Can you work these out from the model? Positions are in its coordinate system, mm. A direction names the side the tool comes from. Give positions to 0.01 mm unless a question says otherwise; leave off trailing zeros. Loops run counter-clockwise (first coordinate to the right, second up) from the corner with the lowest first, then second, coordinate; pieces in that order, holes last. Notation, with made-up numbers: M 79.25,18.25 L 109.25,18.25 A14 cw 109.25,29.25 Z; hole C 41.5,-12 d6. An arc over 180 degrees is marked long. Put each result on its own line as item: value. Start each with the question number.
1) For P1, Ø5, axis at y = 159.5, z = 3.5, coming from the -X side; P2, Ø2, axis at x = -6, z = -2.5, coming from the +Y side; P3, Ø1.5, axis at x = -5.5, y = 27.5, coming from the +Z side, each with a flat end and sliding along its axis, tell me the tip position at first contact or that it passes through.
2) Imagine slicing it at A-A (x = 0). Write out the boundary of the cut face in (y, z).
3) For faces 1 (the cylindrical face through (-2, 182, 0)), 2 (the flat face through (0, 0, 0)), 3 (the cylindrical face through (1.802, 73.95, 5.723)), which set-ups out of +Z, -Z, +X, -X, +Y, -Y let a thin tool reach every point of the face, with its end or its side?
4) Imagine slicing it at B-B (z = 0). Write out the boundary of the cut face in (x, y), then the cut area to 3 significant figures.
5) Imagine slicing it at C-C (y = 59). Write out the boundary of the cut face in (x, z), then the cut area to 3 significant figures.
6) Please list where these lines run through material, in increasing order: line 1 along Y through (x, z) = (3, 3.75); line 2 along Y through (x, z) = (0, 6.5); line 3 along X through (y, z) = (123, 0.5). Write a range as from..to.
from build123d import *

# Parameters (mm, degrees)
SKETCH1_R            = 6
ELECTRODE_BODY_DEPTH = 150
CAP_START            = 150
SKETCH2_R            = 8
CAP_DEPTH            = 25
CABLE_STUB_START     = 175
SKETCH3_R            = 2
CABLE_STUB_DEPTH     = 15
SKETCH4_R            = 2
PLATINUM_TIP_DEPTH   = 1.5


with BuildPart() as part:
    # Sketch1 → Electrode_Body (new body)
    with BuildSketch(Plane(origin=(0, 0, 0), x_dir=(1, 0, 0), z_dir=(0, 1, 0))):
        with Locations(Location((0, 0, 0), (0, 0, 270))):
            Circle(SKETCH1_R)
    extrude(amount=ELECTRODE_BODY_DEPTH)

    # Sketch2 → Cap (add)
    with BuildSketch(Plane(origin=(0, 0, 0), x_dir=(1, 0, 0), z_dir=(0, 1, 0)).offset(CAP_START)):
        with Locations(Location((0, 0, 0), (0, 0, 270))):
            Circle(SKETCH2_R)
    extrude(amount=CAP_DEPTH)

    # Sketch3 → Cable_Stub (add)
    with BuildSketch(Plane(origin=(0, 0, 0), x_dir=(1, 0, 0), z_dir=(0, 1, 0)).offset(CABLE_STUB_START)):
        with Locations(Location((0, 0, 0), (0, 0, 270))):
            Circle(SKETCH3_R)
    extrude(amount=CABLE_STUB_DEPTH)

    # Sketch4 → Platinum_Tip (add)
    with BuildSketch(Plane(origin=(0, 0, 0), x_dir=(1, 0, 0), z_dir=(0, 1, 0))):
        with Locations(Location((0, 0, 0), (0, 0, 270))):
            Circle(SKETCH4_R)
    extrude(amount=PLATINUM_TIP_DEPTH)


solid = part.part
Recorded:
1. P1: x = -7.94
1. P2: y = 175
1. P3: z = 3.67
2. outline: M 0,-6 L 150,-6 L 150,-8 L 175,-8 L 175,-2 L 190,-2 L 190,2 L 175,2 L 175,8 L 150,8 L 150,6 L 0,6 Z
3. face 1: +Y
3. face 2: +Z, -Z, +X, -X, -Y
3. face 3: -Y
4. outline: M -8,150 L -6,150 L -6,0 L 6,0 L 6,150 L 8,150 L 8,175 L 2,175 L 2,190 L -2,190 L -2,175 L -8,175 Z
4. area: 2,260 mm²
5. outline: C 0,0 d12
5. area: 113 mm²
6. line 1: 0..175
6. line 2: 150..175
6. line 3: -5.98..5.98
